Can you work these out from the model? Positions are in its coordinate system, mm. Face numbers are marked on the shaded views. A direction names the side the tool comes from. Coordinates: 2 decimals unless noted, no trailing zeros. Loops run counter-clockwise (first coordinate to the right, second up) from the corner with the lowest first, then second, coordinate; pieces in that order, holes last.
```python
from build123d import *

# Parameters (mm, degrees)
SKETCH1_W               = 12.5
SKETCH1_H               = 5.2
BOSS_EXTRUDE1_DEPTH     = 2
SKETCH2_W               = 7.8
SKETCH2_H               = 2
CUT_EXTRUDE1_DEPTH      = 2.7
SKETCH3_W               = 10
SKETCH3_H               = 2.5
BOSS_EXTRUDE2_DEPTH     = 4.6
SKETCH4_W               = 10
SKETCH4_H               = 3.5
BOSS_EXTRUDE3_DEPTH     = 28.7
SKETCH5_W               = 10
SKETCH5_H               = 8
BOSS_EXTRUDE4_DEPTH     = 2
CUT_EXTRUDE2_DEPTH      = 37.730811317
CUT_EXTRUDE2_DEPTH_BACK = 37.730811317
SKETCH6_W               = 5
SKETCH6_H               = 2
SKETCH7_W               = 15.5
SKETCH7_H               = 6.7
SKETCH7_W_2             = 7.8
SKETCH7_H_2             = 2.7
BOSS_EXTRUDE5_DEPTH     = 1
CHAMFER1_SIZE           = 0.5


with BuildPart() as part:
    # Sketch1 → Boss-Extrude1 (new body)
    with BuildSketch(Plane.XY):
        with Locations((0, 2.6)):
            Rectangle(SKETCH1_W, SKETCH1_H)
    extrude(amount=BOSS_EXTRUDE1_DEPTH)

    # Sketch2 → Cut-Extrude1 (cut)
    with BuildSketch(Plane(origin=(0, 5.2, 0), x_dir=(1, 0, 0), z_dir=(0, 1, 0))):
        with Locations((0, -1)):
            Rectangle(SKETCH2_W, SKETCH2_H)
    extrude(amount=-CUT_EXTRUDE1_DEPTH, mode=Mode.SUBTRACT)

    # Sketch3 → Boss-Extrude2 (add)
    with BuildSketch(Plane(origin=(0, 0, 0), x_dir=(-1, 0, 0), z_dir=(0, 0, -1))):
        with Locations((0, 1.25)):
            Rectangle(SKETCH3_W, SKETCH3_H)
    extrude(amount=BOSS_EXTRUDE2_DEPTH)

    # Sketch4 → Boss-Extrude3 (add)
    with BuildSketch(Plane(origin=(0, 0, -4.6), x_dir=(-1, 0, 0), z_dir=(0, 0, -1))):
        with Locations((0, 1.75)):
            Rectangle(SKETCH4_W, SKETCH4_H)
    extrude(amount=BOSS_EXTRUDE3_DEPTH)

    # Sketch5 → Boss-Extrude4 (add)
    with BuildSketch(Plane(origin=(0, 0, -33.3), x_dir=(-1, 0, 0), z_dir=(0, 0, -1))):
        with Locations((0, 4)):
            Rectangle(SKETCH5_W, SKETCH5_H)
    extrude(amount=BOSS_EXTRUDE4_DEPTH)

    # Sketch6 → Cut-Extrude2 (cut, two sides: drawn at the far end of the back side and taken through both)
    with BuildSketch(Plane(origin=(0, 0, 0), x_dir=(0, 0, -1), z_dir=(1, 0, 0)).offset(-CUT_EXTRUDE2_DEPTH_BACK)):
        with Locations((11.5, 2.698552558)):
            Rectangle(SKETCH6_W, SKETCH6_H)
    extrude(amount=CUT_EXTRUDE2_DEPTH + CUT_EXTRUDE2_DEPTH_BACK, mode=Mode.SUBTRACT)

    # Sketch7 → Boss-Extrude5 (add)
    with BuildSketch(Plane.XY.offset(2)):
        with Locations((0, 3.35)):
            Rectangle(SKETCH7_W, SKETCH7_H)
        with Locations((0, 3.85)):
            Rectangle(SKETCH7_W_2, SKETCH7_H_2, mode=Mode.SUBTRACT)
    extrude(amount=BOSS_EXTRUDE5_DEPTH)

    # Chamfer1
    chamfer1_edges = [part.edges().sort_by_distance(p)[0] for p in [
        (0, 5.2, 3),
        (-7.75, 3.35, 3),
        (0, 0, 3),
        (7.75, 3.35, 3),
        (0, 6.7, 3),
        (-3.9, 3.85, 3),
        (0, 2.5, 3),
        (3.9, 3.85, 3),
    ]]
    chamfer(chamfer1_edges, length=CHAMFER1_SIZE)


solid = part.part
```
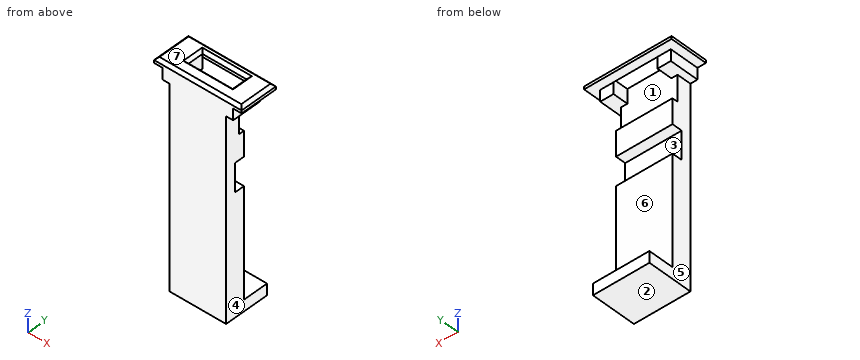
(1) I want a section at B-B on x = 3. Write out the boundary of the cut face in (y, z).
Check values:
outline: (0, -35.3) - (8, -35.3) - (8, -33.3) - (3.5, -33.3) - (3.5, -14) - (1.7, -14) - (1.7, -9) - (3.5, -9) - (3.5, -4.6) - (2.5, -4.6) - (2.5, 2.5) - (2, 3) - (0.5, 3) - (0, 2.5) - close; (5.2, 2) - (6.7, 2) - (6.7, 2.5) - (6.2, 3) - (5.7, 3) - (5.2, 2.5) - close
(2) Which directions (+Z, -Z, +X, -X, +Y, -Y) give clear straight access to the entire face, cutting with the end or side of a thin tool? Please do the marked faces 5, 6 and 7.
Check values:
face 5: -Z, -X, +Y, -Y
face 6: +X, -X, +Y
face 7: +Z, +X, -X, +Y, -Y
(3) I'm going to push flat-ended pins straight in: pin 1 (3.5 mm diameter, centred on x = 1.5, y = 5.5, fed in from +Z); pin 2 (0.8 mm diameter, centred on y = 3.5, z = 1.5, fed in from -X); pin 3 (3 mm diameter, centred on x = -0.5, z = -19, fed in from +Y); pin 4 (1.6 mm diameter, centred on x = -5.5, z = 1, fed in from +Y). Where does each tip first touch, or does it pass through?
Check values:
pin 1: stops at z = 3
pin 2: stops at x = -6.25
pin 3: stops at y = 3.5
pin 4: stops at y = 5.2
(4) I want a section at C-C on y = 1. Write out the boundary of the cut face in (x, z), then the cut area to 3 significant figures.
Check values:
outline: (-7.75, 2) - (-6.25, 2) - (-6.25, 0) - (-5, 0) - (-5, -35.3) - (5, -35.3) - (5, 0) - (6.25, 0) - (6.25, 2) - (7.75, 2) - (7.75, 2.5) - (7.25, 3) - (-7.25, 3) - (-7.75, 2.5) - close
area: 393 mm2
(5) If I drill on probe 1 along X at (y, z) = (3, 1); probe 2 along Z at (x, y) = (-3, 3); probe 3 along Z at (x, y) = (1, 6), over which ranges is the centre line in solid material (lowest first)?
Check values:
probe 1: x = -6.25 to -3.9, 3.9 to 6.25
probe 2: z = -35.3 to -14, -9 to -4.6
probe 3: z = -35.3 to -33.3, 2 to 3
(6) I want a section at A-A on y = 4.25. Write out the boundary of the cut face in (x, z).
Check values:
outline: (-7.75, 2) - (-6.25, 2) - (-6.25, 0) - (-3.9, 0) - (-3.9, 2.5) - (-4.4, 3) - (-7.25, 3) - (-7.75, 2.5) - close; (-5, -35.3) - (5, -35.3) - (5, -33.3) - (-5, -33.3) - close; (3.9, 0) - (6.25, 0) - (6.25, 2) - (7.75, 2) - (7.75, 2.5) - (7.25, 3) - (4.4, 3) - (3.9, 2.5) - close
(7) If we mould it in two halves opening along Z, with no side actions, what happens to the marked faces 1, 2, 3 and 4? For each: released by +Z, released by -Z, zero draft, split by the parting line, or undercut.
Check values:
face 1: undercut
face 2: released by -Z
face 3: undercut
face 4: zero draft
(8) I want a section at D-D on z = -3. Write out the boundary of the cut face in (x, y).
Check values:
outline: (-5, 0) - (5, 0) - (5, 2.5) - (-5, 2.5) - close
